Autodesk Inventor part; units mm, degrees
ref_plane "YZ Plane" through (0, 0, 0) normal (1, 0, 0) x (0, 1, 0)
ref_plane "XZ Plane" through (0, 0, 0) normal (0, 1, 0) x (-1, 0, 0)
ref_plane "XY Plane" through (0, 0, 0) normal (0, 0, 1) x (1, 0, 0)
sketch "Sketch1" plane through (0, 0, 0) normal (1, 0, 0) x (0, 1, 0)
  line L0 (0, 0) -> (60, 0)
  line L1 (60, 0) -> (60, 60)
  line L2 (60, 60) -> (0, 60)
  line L3 (0, 60) -> (0, 0)
  line L4 (60, 60) -> (40, 60) construction
  line L5 (40, 60) -> (40, 40) construction
  line L6 (40, 40) -> (60, 40) construction
  line L7 (60, 40) -> (60, 60) construction
  line L8 (40, 40) -> (60, 40) construction
  line L9 (60, 40) -> (60, 20) construction
  line L10 (60, 20) -> (40, 20) construction
  line L11 (40, 20) -> (40, 40) construction
  line L12 (40, 20) -> (60, 20) construction
  line L13 (60, 20) -> (60, 0) construction
  line L14 (60, 0) -> (40, 0) construction
  line L15 (40, 0) -> (40, 20) construction
  line L16 (40, 20) -> (20, 20) construction
  line L17 (20, 20) -> (20, 0) construction
  line L18 (20, 0) -> (40, 0) construction
  line L19 (40, 0) -> (40, 20) construction
  line L20 (20, 20) -> (40, 20) construction
  line L21 (40, 20) -> (40, 40) construction
  line L22 (40, 40) -> (20, 40) construction
  line L23 (20, 40) -> (20, 20) construction
  line L24 (40, 40) -> (20, 40) construction
  line L25 (20, 40) -> (20, 60) construction
  line L26 (20, 60) -> (40, 60) construction
  line L27 (40, 60) -> (40, 40) construction
  line L28 (20, 60) -> (0, 60) construction
  line L29 (0, 60) -> (0, 40) construction
  line L30 (0, 40) -> (20, 40) construction
  line L31 (20, 40) -> (20, 60) construction
  line L32 (0, 40) -> (20, 40) construction
  line L33 (20, 40) -> (20, 20) construction
  line L34 (20, 20) -> (0, 20) construction
  line L35 (0, 20) -> (0, 40) construction
  line L36 (20, 20) -> (0, 20) construction
  line L37 (0, 20) -> (0, 0) construction
  line L38 (0, 0) -> (20, 0) construction
  line L39 (20, 0) -> (20, 20) construction
  line L40 (60, 10) -> (0, 10) construction
  line L41 (60, 30) -> (0, 30) construction
  line L42 (60, 50) -> (0, 50) construction
  line L43 (50, 60) -> (50, 0) construction
  line L44 (30, 60) -> (30, 0) construction
  line L45 (10, 60) -> (10, 0) construction
  circle A0 centre (50, 50) radius 2.6
  circle A1 centre (50, 30) radius 2.6
  circle A2 centre (50, 10) radius 2.6
  circle A3 centre (30, 10) radius 2.6
  circle A4 centre (30, 30) radius 2.6
  circle A5 centre (30, 50) radius 2.6
  circle A6 centre (10, 50) radius 2.6
  circle A7 centre (10, 30) radius 2.6
  circle A8 centre (10, 10) radius 2.6
  dimension "d0" = 60
  dimension "d1" = 60
  dimension "d2" = 20
  dimension "d3" = 20
  dimension "d4" = 20
  dimension "d5" = 20
  dimension "d6" = 20
  dimension "d7" = 20
  dimension "d8" = 20
  dimension "d9" = 20
  dimension "d10" = 5.2
  dimension "d11" = 5.2
  dimension "d12" = 5.2
  dimension "d13" = 5.2
  dimension "d14" = 5.2
  dimension "d15" = 5.2
  dimension "d16" = 5.2
  dimension "d17" = 5.2
  dimension "d18" = 5.2
extrude "Extrusion1" add sketch "Sketch1" against normal blind 3.175
fillet "Fillet1" radius 3.175 4 edges at (-1.5875, 60, 60) (-1.5875, 0, 60) (-1.5875, 0, 0) (-1.5875, 60, 0)
equation "\"d11\" = d10"
equation "\"d12\" = d10"
equation "\"d13\" = d10"
equation "\"d14\" = d10"
equation "\"d15\" = d10"
equation "\"d16\" = d10"
equation "\"d17\" = d10"
equation "\"d18\" = d10"
properties part number "Generic 3x3 Corner Connecting Gusset"
For this review, take the finished solid that the model builds, in its own axes (mm). Give positions to 0.01 mm unless a question says otherwise; leave off trailing zeros. Loops run counter-clockwise (first coordinate to the right, second up) from the corner with the lowest first, then second, coordinate; pieces in that order, holes last.
Item 1: Take a section at C-C, the plane x = -1.75. Give the number of separate pieces and of enclosed holes in the cut face, and give its area (3 significant figures).
Item 2: For line 1 along Z through (x, y) = (-1.4, 10); line 2 along Z through (x, y) = (-1.95, 49), list the stretches that pass through material, from the lowest coordinate up.
Item 3: Draft analysis for pull direction Z (two halves, no side actions). For faces 1 (the flat face through (0, 30, 24)), 2 (the flat face through (-2, 30, 60)), 3 (the cylindrical face through (-1.6, 47.4, 30.1)), state which applies: +Z half, -Z half, draft (parallel to the pull), parting line (faces both ways), or undercut.
Item 4: Take a section at A-A, the plane z = 49. State the section outline as (x, y) points (3 decimals), and give its area (3 significant figures).
Calculated:
1. separate pieces: 1
1. enclosed holes: 9
1. area: 3,400 mm2
2. line 1: z = 0 to 7.4, 12.6 to 27.4, 32.6 to 47.4, 52.6 to 60
2. line 2: z = 0 to 7.6, 12.4 to 27.6, 32.4 to 47.6, 52.4 to 60
3. face 1: draft
3. face 2: +Z half
3. face 3: undercut
4. outline: (-3.175, 0) - (0, 0) - (0, 7.6) - (-3.175, 7.6) - close; (-3.175, 12.4) - (0, 12.4) - (0, 27.6) - (-3.175, 27.6) - close; (-3.175, 32.4) - (0, 32.4) - (0, 47.6) - (-3.175, 47.6) - close; (-3.175, 52.4) - (0, 52.4) - (0, 60) - (-3.175, 60) - close
4. area: 145 mm2
